Source: three-view drawing plus pictorial views. Frame: mm from the lowest corner of the part. Give positions to 0.01 mm unless a question says otherwise; leave off trailing zeros. Order: outer loops, then holes, each group sorted by start corner. A loop starts at its lowest first (then second) coordinate and runs counter-clockwise, first axis right, second up. Notation, with made-up numbers: (55, 24.5) - (90, 24.5) arc R10 ccw to (90, 40.5) - close; hole circle Ø10 at (-16.75, -32). An arc over 180 degrees is marked (long way). Answer in a Markdown table with one row per item. Add a question column.
1. Ray query, line 1 (X direction, y = 251, z = 188.5); line 2 (Z direction, x = 1769, y = 26). Return the intervals inside material, ascending. Write a range as [from, to].
2. Mould query, pull axis Z, two halves, no side actions, for the marked faces 1 and 2. Classes: released by +Z, released by -Z, zero draft, split by the parting line, or undercut.
3. Section query B-B on z = 440. Return loops of the section in (x, y), and give its area (3 significant figures).
4. Section query C-C on x = 1867.5. Return loops of the section in (y, z).
5. Section query A-A on y = 348.5. Return loops of the section in (x, z).
6. Contact query for a flat-ended pin moving along its axis: pin 1 (8 mm diameter, centred on y = 385, z = 673.5, fed in from -X). Output: stop coordinate, or through.
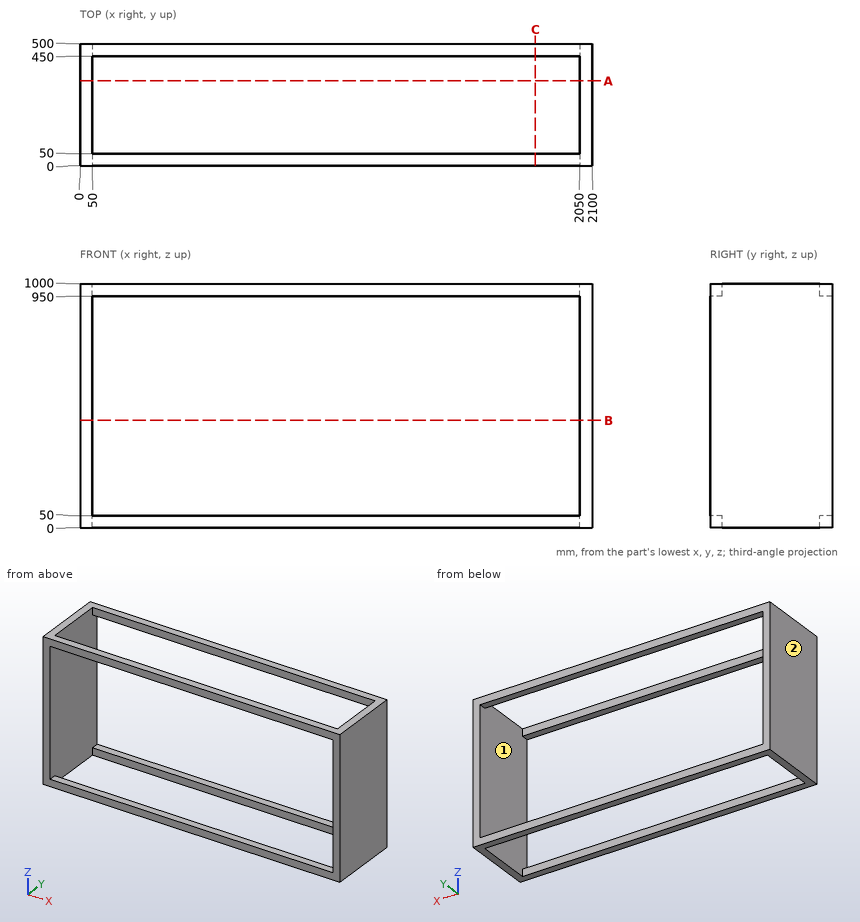
Answer:
| question | item | result |
|---|---|---|
| 1 | line 1 | x = [0, 50], [2050, 2100] |
| 1 | line 2 | z = [0, 50], [950, 1000] |
| 2 | face 1 | undercut |
| 2 | face 2 | zero draft |
| 3 | outline | (0, 0) - (50, 0) - (50, 500) - (0, 500) - close; (2050, 0) - (2100, 0) - (2100, 500) - (2050, 500) - close |
| 3 | area | 50,000 mm² |
| 4 | outline | (0, 0) - (50, 0) - (50, 50) - (0, 50) - close; (0, 950) - (50, 950) - (50, 1000) - (0, 1000) - close; (450, 0) - (500, 0) - (500, 50) - (450, 50) - close; (450, 950) - (500, 950) - (500, 1000) - (450, 1000) - close |
| 5 | outline | (0, 0) - (50, 0) - (50, 1000) - (0, 1000) - close; (2050, 0) - (2100, 0) - (2100, 1000) - (2050, 1000) - close |
| 6 | pin 1 | stops at x = 0 |
